Can you work these out from the drawing? Everything is in mm from the part's minimum corner. Coordinates: 2 decimals unless noted, no trailing zeros. Order: outer loops, then holes, each group sorted by start corner. A loop starts at its lowest first (then second) coordinate and runs counter-clockwise, first axis right, second up. Notation, with made-up numbers: (-14, -5) - (41, -5) arc R24 cw to (41, 27) - close; hole circle Ø6 at (21, 43.5). An arc over 180 degrees is marked (long way). Answer as CSV lines item,"result". Start each with the question number.
Q1. I need wall thicknesses on line 1 (Z direction, x = 3, y = 3.55); line 2 (Y direction, x = 3.25, z = 9.5); line 3 (Y direction, x = 3.7, z = 9.75). Which ranges of each line are inside material? Lowest first, please.
Q2. Suppose I cut it at C-C (z = 7). Please give me the cut outline in (x, y).
Q3. Thinking about a two-plate mould opening in Y: for the marked faces 1, 2 and 3, which applies, released by +Y, released by -Y, zero draft, split by the parting line, or undercut?
Q4. Suppose I cut it at B-B (y = 2.9). Please give me the cut outline in (x, z).
Q5. For pin 1 Ø3 at (x, z) = (2.5, 5.5) entering from -Y; pin 2 Ø1.1 at (y, z) = (2.5, 9.5) entering from -X; pin 3 Ø3 at (y, z) = (3.5, 1.5) entering from -X; pin 4 Ø1 at (x, y) = (5, 2) entering from -Z (1 decimal), each with a flat end and sliding along its axis, tell me the tip position at first contact or that it passes through.
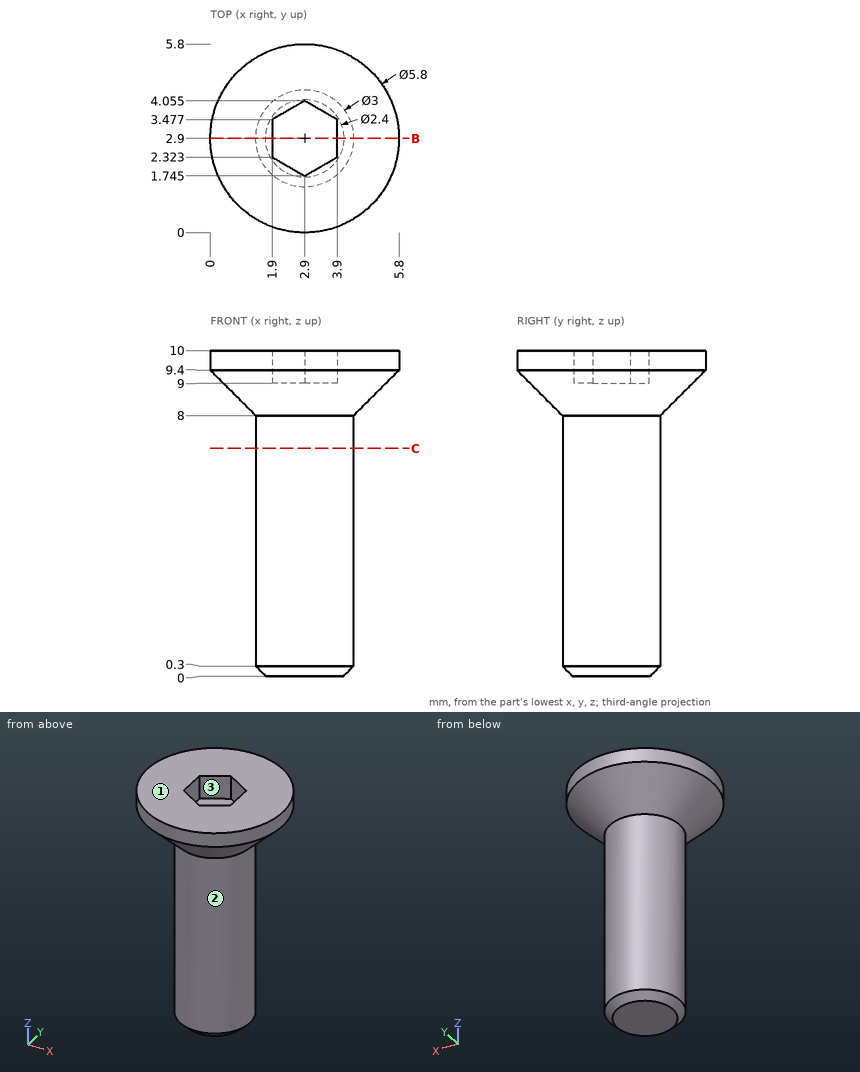
Here are the results:
1,line 1,"z = 0 to 9"
1,line 2,"y = 0.02 to 1.95, 3.85 to 5.78"
1,line 3,"y = 0.11 to 2.21, 3.59 to 5.69"
2,outline,"circle Ø3 at (2.9, 2.9)"
3,face 1,"zero draft"
3,face 2,"split by the parting line"
3,face 3,"undercut"
4,outline,"(0, 9.4) - (1.4, 8) - (1.4, 0.3) - (1.7, 0) - (4.1, 0) - (4.4, 0.3) - (4.4, 8) - (5.8, 9.4) - (5.8, 10) - (3.9, 10) - (3.9, 9) - (1.9, 9) - (1.9, 10) - (0, 10) - close"
5,pin 1,"stops at y = 1.4"
5,pin 2,"stops at x = 0"
5,pin 3,"stops at x = 1.4"
5,pin 4,"stops at z = 8.3"
